Input: part model. Units: mm. Frame: model coordinates. Face numbers are marked on the shaded views. Give positions to 0.01 mm unless a question says otherwise; leave off trailing zeros. Loops run counter-clockwise (first coordinate to the right, second up) from the corner with the lowest first, then second, coordinate; pieces in that order, holes last. Notation, with made-up numbers: (89, 81.25) - (124, 81.25) arc R15 ccw to (124, 106.25) - close; hole circle Ø1 at (34.25, 32). An arc over 180 degrees is marked (long way). One line per question, with ' | ' between items. Start each with the question number.
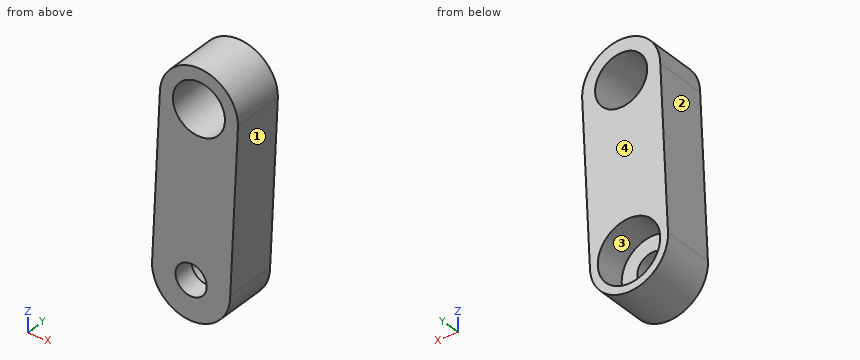
Autodesk Inventor part; units mm, degrees
ref_plane "YZ Plane" through (0, 0, 0) normal (1, 0, 0) x (0, 1, 0)
ref_plane "XZ Plane" through (0, 0, 0) normal (0, 1, 0) x (-1, 0, 0)
ref_plane "XY Plane" through (0, 0, 0) normal (0, 0, 1) x (1, 0, 0)
sketch "Sketch1" plane through (0, 0, 0) normal (0, 1, 0) x (-1, 0, 0)
  circle A0 centre (-0.749959, 8.455141) radius 2.5
  circle A1 centre (0, -7.527273) radius 1.5
  circle A2 centre (-0.749959, 8.455141) radius 3.75
  circle A3 centre (0, -7.527273) radius 3
  line L0 (3, 8.472727) -> (3, -7.527273)
  line L1 (-4.499959, 8.455141) -> (-2.987099, -7.805192)
  circle A4 centre (0, -7.527273) radius 3.75
  line L2 (-4.499959, 8.455141) -> (-3.75, -7.527273)
  line L3 (3, 8.472727) -> (3.745841, -7.350712)
  point P0 (0, 0)
  dimension "d0" = 16
  dimension "d1" = 5
  dimension "d2" = 3
  dimension "d3" = 7.5
  dimension "d4" = 6
  dimension "d10" = 7.5
sketch "Sketch1 outline for Extrusion1" plane through (0, 0, 0) normal (0, 1, 0) x (-1, 0, 0)
  arc A0 (3, 8.472727) -> (-4.499959, 8.455141) centre (-0.749959, 8.455141) ccw
  line L0 (-4.499959, 8.455141) -> (-3.75, -7.527273)
  arc A1 (-3.75, -7.527273) -> (3.745841, -7.350712) centre (0, -7.527273) ccw
  line L1 (3.745841, -7.350712) -> (3, 8.472727)
  circle A2 centre (0, -7.527273) radius 1.5
  circle A3 centre (-0.749959, 8.455141) radius 2.5
extrude "Extrusion1" add sketch "Sketch1 outline for Extrusion1" along normal blind 5
sketch "Sketch2" plane through (0, 5, 0) normal (0, 1, 0) x (1, 0, 0)
  circle A0 centre (0, 7.527273) radius 1.5
  circle A1 centre (0, 7.527273) radius 3
  point P0 (0, 0)
  point P1 (3, 7.527273)
  dimension "d7" = 6
extrude "Extrusion2" cut sketch "Sketch2" against normal blind 3
sketch "Sketch3" plane through (0, 5, 0) normal (0, 1, 0) x (1, 0, 0)
  circle A0 centre (0.749959, -8.455141) radius 2.5
  circle A1 centre (0, 7.527273) radius 3
  circle A2 centre (0, 7.527273) radius 1.5
  arc A3 (3.75, 7.527273) -> (-3.745841, 7.350712) centre (0, 7.527273) ccw
  point P0 (0, 0)
properties part number "Redesign_Linkage_3DPrint"
Q1. Line query: L1, parallel to Z at x = 1.25, y = 2.9; L2, parallel to Z at x = 0, y = 1.2; L3, parallel to Y at x = -0.75, z = -6. Output: solid intervals per line, ascending. Write a range as from..to.
Q2. Section D-D, the plane y = 0.7. Output: boundary loops of the cut face in (x, z).
Q3. Section B-B, the plane y = 4.15. Output: boundary loops of the cut face in (x, z).
Q4. First-contact query: pin 1 (1.8 mm diameter, centred on x = 0.5, z = -8, fed in from +Y); pin 2 (3 mm diameter, centred on y = 2.5, z = -8, fed in from +X); pin 3 (2 mm diameter, centred on y = 3.5, z = -6, fed in from -X). Flat tips, straight axial feed; report the tip coordinate or a pass-through.
Q5. Section C-C, the plane z = -7.75. Output: boundary loops of the cut face in (x, y), plus the area to 4 significant figures.
Q6. Section A-A, the plane x = 0. Output: boundary loops of the cut face in (y, z), plus the area to 3 significant figures.
Q7. Draft query along X for the marked faces 1, 2, 3 and 4. Return one class per face: +X half, -X half, draft (parallel to the pull), parting line (faces both ways), or undercut.
Solved:
1) L1: z = -11.06..-10.25, -4.8..6.01, 10.9..12.17 | L2: z = -11.28..-9.03, -6.03..6.07, 10.84..12.13 | L3: y = 0..2
2) outline: (-3.75, -7.35) arc R3.75 ccw (long way) to (3.75, -7.53) - (4.5, 8.46) arc R3.75 ccw to (-3, 8.47) - close; hole circle Ø5 at (0.75, 8.46); hole circle Ø3 at (0, -7.53)
3) outline: (-3.75, -7.35) arc R3.75 ccw (long way) to (3.75, -7.53) - (4.5, 8.46) arc R3.75 ccw to (-3, 8.47) - close; hole circle Ø6 at (0, -7.53); hole circle Ø5 at (0.75, 8.46)
4) pin 1: stops at y = 2 | pin 2: stops at x = 3.8 | pin 3: stops at x = -3.73
5) outline: (-3.74, 0) - (-1.48, 0) - (-1.48, 2) - (-2.99, 2) - (-2.99, 5) - (-3.74, 5) - close; (1.48, 0) - (3.74, 0) - (3.74, 5) - (2.99, 5) - (2.99, 2) - (1.48, 2) - close | area: 13.55 mm²
6) outline: (0, -11.28) - (5, -11.28) - (5, -10.53) - (2, -10.53) - (2, -9.03) - (0, -9.03) - close; (0, -6.03) - (2, -6.03) - (2, -4.53) - (5, -4.53) - (5, 6.07) - (0, 6.07) - close; (0, 10.84) - (5, 10.84) - (5, 12.13) - (0, 12.13) - close | area: 69.2 mm²
7) face 1: +X half | face 2: -X half | face 3: undercut | face 4: draft
